Check sheet for the modelled part. Datum: model origin and axes. Units: mm. A direction names the side the tool comes from. Coordinates: 2 decimals unless noted, no trailing zeros. Loops run counter-clockwise (first coordinate to the right, second up) from the corner with the lowest first, then second, coordinate; pieces in that order, holes last. Notation, with made-up numbers: (77, 8.5) - (126, 8.5) arc R15 ccw to (126, 36.5) - close; hole circle Ø10 at (50.5, -17.75). An arc over 180 degrees is marked (long way). Use a Markdown table: item, result. Add a question column.
1) Tool access check on faces 4 (the flat face through (74, 5.1, -4)), 5 (the cylindrical face through (16, 17.9, -7)), 6 (the flat face through (74, 31.6, -4)), 7 (the flat face through (74, 23, -7.5)). Record the directions out of +Z, -Z, +X, -X, +Y, -Y that give a thin tool (end or side, any length) a straight path to the whole face; none if there is none.
2) Draft check along Y on faces 1 (the flat face through (74, 2, -1)), 2 (the cylindrical face through (124, 17.8, -7)), 3 (the flat face through (74, 4.1, -4)). Enter one of: pulls with the +Y half, pulls with the -Y half, needs draft (parallel to the pull), parting line crosses it, or undercut.
3) Sectioned sample at C-C, the plane y = 25. Enter the section's corners in (x, z), then the cut area to 3 significant figures.
4) Thickness scan on line 1 (Y direction, x = 10.5, z = -5); line 2 (Z direction, x = 87, y = 9); line 3 (Y direction, x = 91.5, z = -0.25). Record the ranges inside material, lowest first.
5) Sectioned sample at A-A, the plane y = 17.85. State how many separate pieces and enclosed holes the cut face has, then the cut area to 3 significant figures.
6) Sectioned sample at B-B, the plane x = 39. Enter the section's corners in (y, z), then the cut area to 3 significant figures.
7) Go/stop test with flat-tipped pins: P1, Ø2.5, axis at x = 58, y = 34, coming from the -Z side; P2, Ø3, axis at x = 79, z = -6, coming from the -Y side; P3, Ø0.8, axis at x = 131, z = -7, coming from the +Y side. Record where each tip stops, or that it passes through.
from build123d import *

# Parameters (mm, degrees)
BOSS_EXTRUDE1_DEPTH = 150
CUT_EXTRUDE1_DEPTH  = 155.372082968
LPATTERN1_COUNT     = 8
LPATTERN1_PITCH     = 20
FILLET1_R           = 2


with BuildPart() as part:
    # Sketch1 → Boss-Extrude1 (new body)
    with BuildSketch(Plane(origin=(0, 0, 0), x_dir=(0, 0, -1), z_dir=(1, 0, 0))):
        with BuildLine():
            Line((0, 0), (0, 3.1))
            ThreePointArc((0, 3.1), (0.585786438, 4.514213562), (2, 5.1))
            Line((2, 5.1), (5.5, 5.1))
            ThreePointArc((5.5, 5.1), (6.207106781, 5.392893219), (6.5, 6.1))
            Line((6.5, 6.1), (6.5, 29.6))
            ThreePointArc((6.5, 29.6), (6.207106781, 30.307106781), (5.5, 30.6))
            Line((5.5, 30.6), (2, 30.6))
            ThreePointArc((2, 30.6), (0.585786438, 31.185786438), (0, 32.6))
            Line((0, 32.6), (0, 35.7))
            Line((0, 35.7), (1, 35.7))
            Line((1, 35.7), (1, 32.6))
            ThreePointArc((1, 32.6), (1.292893219, 31.892893219), (2, 31.6))
            Line((2, 31.6), (5.5, 31.6))
            ThreePointArc((5.5, 31.6), (6.914213562, 31.014213562), (7.5, 29.6))
            Line((7.5, 29.6), (7.5, 6.1))
            ThreePointArc((7.5, 6.1), (6.914213562, 4.685786438), (5.5, 4.1))
            Line((5.5, 4.1), (2, 4.1))
            ThreePointArc((2, 4.1), (1.292893219, 3.807106781), (1, 3.1))
            Line((1, 3.1), (1, 0))
            Line((1, 0), (0, 0))
        make_face()
    extrude(amount=BOSS_EXTRUDE1_DEPTH)

    # Sketch2 → Cut-Extrude1 (cut, through all)
    with BuildSketch(Plane.XY):
        with BuildLine():
            Line((7.15, 21), (12.85, 21))
            ThreePointArc((12.85, 21), (16, 17.85), (12.85, 14.7))
            Line((12.85, 14.7), (7.15, 14.7))
            ThreePointArc((7.15, 14.7), (4, 17.85), (7.15, 21))
        make_face()
    cut_extrude1 = extrude(amount=-CUT_EXTRUDE1_DEPTH, mode=Mode.SUBTRACT)

    # LPattern1: Cut-Extrude1 ×8
    with Locations(*[(i * LPATTERN1_PITCH, 0, 0) for i in range(1, LPATTERN1_COUNT)]):
        add(cut_extrude1, mode=Mode.SUBTRACT)

    # Fillet1
    fillet1_edges = [part.edges().sort_by_distance(p)[0] for p in [
        (0, 35.7, -0.5),
        (0, 0, -0.5),
        (150, 35.7, -0.5),
        (150, 0, -0.5),
    ]]
    fillet(fillet1_edges, radius=FILLET1_R)


solid = part.part
Solved:
| question | item | result |
|---|---|---|
| 1 | face 4 | +Z, +X, -X |
| 1 | face 5 | +Z, -Z |
| 1 | face 6 | -Z, +X, -X, +Y |
| 1 | face 7 | -Z, +X, -X, +Y, -Y |
| 2 | face 1 | needs draft |
| 2 | face 2 | undercut |
| 2 | face 3 | pulls with the -Y half |
| 3 | outline | (0, -7.5) - (150, -7.5) - (150, -6.5) - (0, -6.5) - close |
| 3 | area | 150 mm2 |
| 4 | line 1 | y = 4.1 to 5.1, 30.6 to 31.6 |
| 4 | line 2 | z = -7.5 to -6.5 |
| 4 | line 3 | y = 0 to 4.07, 31.63 to 35.7 |
| 5 | separate pieces | 8 |
| 5 | enclosed holes | 0 |
| 5 | area | 60.0 mm2 |
| 6 | outline | (0, -1) - (3.1, -1) arc R1 cw to (4.1, -2) - (4.1, -5.5) arc R2 ccw to (6.1, -7.5) - (29.6, -7.5) arc R2 ccw to (31.6, -5.5) - (31.6, -2) arc R1 cw to (32.6, -1) - (35.7, -1) - (35.7, 0) - (32.6, 0) arc R2 ccw to (30.6, -2) - (30.6, -5.5) arc R1 cw to (29.6, -6.5) - (6.1, -6.5) arc R1 cw to (5.1, -5.5) - (5.1, -2) arc R2 ccw to (3.1, 0) - (0, 0) - close |
| 6 | area | 46.1 mm2 |
| 7 | P1 | stops at z = -1 |
| 7 | P2 | stops at y = 4.1 |
| 7 | P3 | stops at y = 31.27 |
